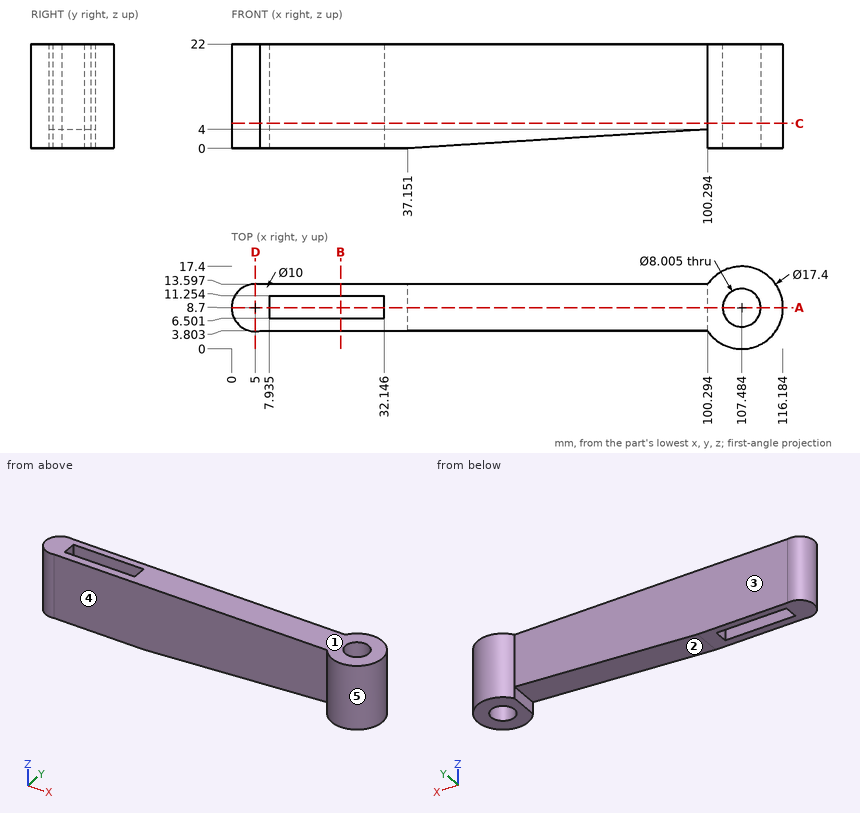
Check sheet for the drawn part. Datum: minimum x, y, z corner. Units: mm. A direction names the side the tool comes from. Round coordinates to 2 decimals unless told otherwise and drop trailing zeros. Loops run counter-clockwise (first coordinate to the right, second up) from the corner with the lowest first, then second, coordinate; pieces in that order, holes last. Notation, with made-up numbers: (5.25, 20) - (18.25, 20) arc R20 ccw to (18.25, 33) - close; hole circle Ø6 at (69, 56). An arc over 180 degrees is marked (long way). Write item = value, one per line. Start each with the question number.
1. Section check A-A on y = 8.7. Give the number of separate pieces and of enclosed holes in the cut face, then the cut area to 3 significant figures.
2. Mould release check, pull along X, two halves, no side actions. Record for the marked faces 1, 2 and 3: released by +X, released by -X, zero draft, split by the parting line, or undercut.
3. Set-up check for the marked faces 4 and 5: record each of +Z, -Z, +X, -X, +Y, -Y from which the full face is reachable in a straight line by a thin tool's end or side.
4. Section check B-B on x = 23. Enter the section's corners in (y, z) (1 decimal), then the cut area to 3 significant figures.
5. Section check C-C on z = 5.25. Enter the section's corners in (x, y) (1 decimal).
6. Thickness scan on line 1 (X direction, y = 8.7, z = 5.5) (1 decimal); line 2 (Y direction, x = 17, z = 9) (1 decimal); line 3 (Y direction, x = 72, z = 8.5). Record the ranges inside material, lowest first.
7. Depth check by flat-ended pin: pin 1 (5 mm diameter, centred on x = 52.5, z = 15.5, fed in from +Y); pin 2 (1.4 mm diameter, centred on y = 9, z = 6, fed in from -X); pin 3 (8 mm diameter, centred on x = 19, z = 3.5, fed in from -Y); pin 4 (3 mm diameter, centred on y = 3.5, z = 9, fed in from +X). Enter the tip coordinate at first touch or a pass-through.
8. Section check D-D on x = 5. Enter the section's corners in (y, z).
Working result:
q1.separate_pieces = 3
q1.enclosed_holes = 0
q1.area = 1,720 mm^2
q2.face_1 = zero draft
q2.face_2 = undercut
q2.face_3 = undercut
q3.face_4 = +Z, -Z, -Y
q3.face_5 = +Z, -Z
q4.outline = (3.8, 0) - (6.5, 0) - (6.5, 22) - (3.8, 22) - close; (11.3, 0) - (13.6, 0) - (13.6, 22) - (11.3, 22) - close
q4.area = 111 mm^2
q5.outline = (6, 3.8) - (100.3, 3.8) arc R8.7 ccw (long way) to (100.3, 13.6) - (6, 13.6) arc R5 ccw (long way) to start; hole (7.9, 6.5) - (32.1, 6.5) - (32.1, 11.3) - (7.9, 11.3) - close; hole circle Ø8 at (107.5, 8.7)
q6.line_1 = 0 to 7.9, 32.1 to 103.5, 111.5 to 116.2
q6.line_2 = 3.8 to 6.5, 11.3 to 13.6
q6.line_3 = 3.8 to 13.6
q7.pin_1 = 13.6
q7.pin_2 = 0
q7.pin_3 = 3.8
q7.pin_4 = 115.36
q8.outline = (3.7, 0) - (13.7, 0) - (13.7, 22) - (3.7, 22) - close
